Design review of the part built by this model. Coordinates are the model's own, in mm. A direction names the side the tool comes from. Coordinates: 2 decimals unless noted, no trailing zeros. Write each loop counter-clockwise with the first axis right and the second up, starting at its lowest first coordinate (ties: lowest second). Pieces come first, ordered by that corner, then holes. Notation, with made-up numbers: (87.5, 43.25) -> (140.5, 43.25) arc R22 ccw to (140.5, 58.25) -> close; hole circle Ø2 at (31.25, -38). An arc over 180 degrees is marked (long way). Write item = value, one per line. Start each with the question number.
```python
from build123d import *

# Parameters (mm, degrees)
CROQUIS1_W                 = 12.8
CROQUIS1_H                 = 12.8
CROQUIS1_W_2               = 10.92
CROQUIS1_H_2               = 10.92
EXTRUIR_L_MINA1_DEPTH      = 280
CORTAR_EXTRUIR1_DEPTH      = 10
CORTAR_EXTRUIR1_DEPTH_BACK = 10
CROQUIS2_R                 = 1.55
CORTAR_EXTRUIR2_DEPTH      = 10
CORTAR_EXTRUIR5_DEPTH      = 10


with BuildPart() as part:
    # Croquis1 → Extruir-L_mina1 (new body)
    with BuildSketch(Plane.XY):
        Rectangle(CROQUIS1_W, CROQUIS1_H)
        Rectangle(CROQUIS1_W_2, CROQUIS1_H_2, mode=Mode.SUBTRACT)
    extrude(amount=-EXTRUIR_L_MINA1_DEPTH)

    # Croquis2 → Cortar-Extruir1 (cut, two sides: drawn at the far end of the back side and taken through both)
    with BuildSketch(Plane(origin=(0, 0, 0), x_dir=(1, 0, 0), z_dir=(0, 1, 0)).offset(-CORTAR_EXTRUIR1_DEPTH_BACK)):
        with Locations(Location((0, 275.11, 0), (0, 0, 180))):
            Circle(CROQUIS2_R)
        with Locations(Location((0, 4.89, 0), (0, 0, 180))):
            Circle(CROQUIS2_R)
    extrude(amount=CORTAR_EXTRUIR1_DEPTH + CORTAR_EXTRUIR1_DEPTH_BACK, mode=Mode.SUBTRACT)

    # Croquis2_3 → Cortar-Extruir2 (cut)
    with BuildSketch(Plane(origin=(0, 0, 0), x_dir=(1, 0, 0), z_dir=(0, 1, 0))):
        with BuildLine():
            Line((3, 240), (3, 221))
            ThreePointArc((3, 221), (0, 218), (-3, 221))
            Line((-3, 221), (-3, 240))
            ThreePointArc((-3, 240), (0, 243), (3, 240))
        make_face()
    extrude(amount=CORTAR_EXTRUIR2_DEPTH, mode=Mode.SUBTRACT)

    # Croquis3 → Cortar-Extruir5 (cut)
    with BuildSketch(Plane(origin=(6.4, 0, 0), x_dir=(0, 0, -1), z_dir=(1, 0, 0))):
        with BuildLine():
            Line((13, 3), (32, 3))
            ThreePointArc((32, 3), (35, 0), (32, -3))
            Line((32, -3), (13, -3))
            ThreePointArc((13, -3), (10, 0), (13, 3))
        make_face()
    extrude(amount=-CORTAR_EXTRUIR5_DEPTH, mode=Mode.SUBTRACT)


solid = part.part
```
(1) For pin 1 Ø5 at (x, y) = (-2.5, -4) entering from +Z; pin 2 Ø2.5 at (x, z) = (0, -275.11) entering from -Y, all flat-tipped, find the tip position at first contact; note any pin that passes through.
(2) For line 1 (Z direction, x = 0, y = -6.05); line 2 (X direction, y = 0.25, z = -221), list the stretches that pass through material, from the lowest coordinate up.
(3) Take a section at B-B, the plane z = -210. State the section outline as (x, y) points.
(4) For faces 1 (the face through (-6.4, 0, -138)), 2 (the face through (-5.46, 0, -138)), list the 3-axis set-ups (+Z, -Z, +X, -X, +Y, -Y) from which the entire face can be reached by the end or side of a thin tool; tool diameter is ignored.
(5) Take a section at A-A, the plane y = 0. State the section outline as (x, z) points.
(6) Mouldability with a two-part tool opening along Y and no side actions: class faces 3 (the face through (0, 6.4, -138)), 4 (the face through (0, -6.4, -138)), 5 (the face through (6, 0, -280)), 6 (the face through (0, -5.46, -138)) as pulls with the +Y half, pulls with the -Y half, needs draft (parallel to the pull), parting line crosses it, or undercut.
Report:
q1.pin_1 = 0
q1.pin_2 = through
q2.line_1 = -280 to -276.66, -273.56 to -6.44, -3.34 to 0
q2.line_2 = -6.4 to -5.46, 5.46 to 6.4
q3.outline = (-6.4, -6.4) -> (6.4, -6.4) -> (6.4, 6.4) -> (-6.4, 6.4) -> close; hole (-5.46, -5.46) -> (5.46, -5.46) -> (5.46, 5.46) -> (-5.46, 5.46) -> close
q4.face_1 = +Z, -Z, -X, +Y, -Y
q4.face_2 = +Z, -Z
q5.outline = (-6.4, -280) -> (-5.46, -280) -> (-5.46, 0) -> (-6.4, 0) -> close; (5.46, -280) -> (6.4, -280) -> (6.4, -35) -> (5.46, -35) -> close; (5.46, -10) -> (6.4, -10) -> (6.4, 0) -> (5.46, 0) -> close
q6.face_3 = pulls with the +Y half
q6.face_4 = pulls with the -Y half
q6.face_5 = needs draft
q6.face_6 = undercut
